Read the model definition and answer for the solid it produces. Units are mm, in the model's axes. A direction names the side the tool comes from. Coordinates: 2 decimals unless noted, no trailing zeros. Loops run counter-clockwise (first coordinate to the right, second up) from the corner with the lowest first, then second, coordinate; pieces in that order, holes last. Notation, with made-up numbers: M -12,69 L 15,69 A24 ccw 15,107 Z; hole C 66,-19 d4. An arc over 180 degrees is marked long. One line per item, written item: value. Start each with the question number.
1. The part is cut by section A-A (z = 0). Write down the section's boundary in (x, y), then the cut area to 3 significant figures.
2. Consider probe 1 along Z at (x, y) = (2.3, 0); probe 2 along Z at (x, y) = (8.25, 0); probe 3 along X at (y, z) = (2.5, -1.5). Determine where each line is inside the solid, lowest interval first.
3. For faces 5 (the face through (10.4, -2, 2)), 6 (the face through (0, 3, -6)), determine the directions among +Z, -Z, +X, -X, +Y, -Y from which every point of the face is accessible in a straight line to the end or side of a thin tool.
4. Flat-ended cylindrical pins translate along their axes: pin 1 (6 mm diameter, centred on y = 0, z = -1, fed in from -X); pin 2 (4.5 mm diameter, centred on y = 0, z = 0, fed in from +X); pin 3 (3 mm diameter, centred on x = 1.5, z = -2, fed in from +Y); pin 4 (6 mm diameter, centred on x = 1.5, z = -4.5, fed in from +Y) (3 decimals). Find the tip coordinate at first contact, or state that the pin passes through.
5. Determine the mould class of faces 1 (the face through (6.85, -0.74, 3.32)), 2 (the face through (7.958, -0.867, 3.905)), 3 (the face through (4, -5, -2)), 4 (the face through (10.7, -2.44, 0.54)) for opening direction Z: +Z half, -Z half, draft (parallel to the pull), parting line (faces both ways), or undercut.
6. The part is cut by section C-C (x = 1.5). Write down the section's boundary in (y, z), then the cut area to 3 significant figures.
Autodesk Inventor part; units mm, degrees
ref_plane "YZ Plane" through (0, 0, 0) normal (1, 0, 0) x (0, 1, 0)
ref_plane "XZ Plane" through (0, 0, 0) normal (0, 1, 0) x (-1, 0, 0)
ref_plane "XY Plane" through (0, 0, 0) normal (0, 0, 1) x (1, 0, 0)
sketch "スケッチ1" plane through (0, 0, 0) normal (0, 0, 1) x (1, 0, 0)
  line L0 (0, 0) -> (11, 0)
  line L1 (11, 0) -> (11, 4)
  line L2 (11, 4) -> (4, 4)
  line L3 (4, 4) -> (4, 6.9)
  line L4 (4, 6.9) -> (0, 6.9)
  line L5 (0, 6.9) -> (0, 0)
  dimension "d9" = 8
  dimension "d10" = 13.8
  dimension "d11" = 4
  dimension "d12" = 7
revolve "回転1" add sketch "スケッチ1" angle 360 about axis through (0, 0, 0) along (1, 0, 0)
shell "Shell1" thickness 0.6 removed faces 1 at (0, 1.1832, -1.6579)
sketch "Sketch2" plane through (11, 0, 0) normal (1, 0, 0) x (0, 0, -1)
  circle A0 centre (0, 0) radius 2.5
  dimension "d14" = 5
extrude "Extrusion1" cut sketch "Sketch2" against normal blind 11
fillet "Fillet1" radius 1 2 edges at (4, -6.9, 0) (4, -4, 0)
properties material "Stainless Steel"
Answer block:
1. outline: M 0,-6.9 L 3,-6.9 A1 ccw 4,-5.9 L 4,-5 A1 cw 5,-4 L 11,-4 L 11,-2.5 L 10.4,-2.5 L 10.4,-3.4 L 3.4,-3.4 L 3.4,-6.3 L 0,-6.3 Z; M 0,6.3 L 3.4,6.3 L 3.4,3.4 L 10.4,3.4 L 10.4,2.5 L 11,2.5 L 11,4 L 5,4 A1 cw 4,5 L 4,5.9 A1 ccw 3,6.9 L 0,6.9 Z
1. area: 17.8 mm2
2. probe 1: z = -6.9 to -6.3, 6.3 to 6.9
2. probe 2: z = -4 to -3.4, 3.4 to 4
2. probe 3: x = 10.4 to 11
3. face 5: -X
3. face 6: +Z, -Z, -X, +Y, -Y
4. pin 1: stops at x = 3.4
4. pin 2: passes through
4. pin 3: stops at y = 6.88
4. pin 4: stops at y = 6.735
5. face 1: undercut
5. face 2: parting line
5. face 3: draft
5. face 4: undercut
6. outline: C 0,0 d13.8; hole C 0,0 d12.6
6. area: 24.9 mm2
